```python
from build123d import *

# Parameters (mm, degrees)
F0_W     = 101.6
F0_H     = 50.8
F0_H_2   = 12.7
F0_H_3   = 76.2
F1_DEPTH = 12.7
F2_W     = 50.8
F2_H     = 203.2
F3_DEPTH = 25.4
F4_W     = 12.7
F4_H     = 50.8
F4_H_2   = 76.2
F5_DEPTH = 25.4
F6_W     = 139.7
F6_H     = 44.45
F7_DEPTH = 25.4


with BuildPart() as f1:
    # F0 (on Front) → F1 (new body)
    with BuildSketch(Plane.XZ):
        with Locations((-41.9671071525, -12.46464407)):
            Rectangle(F0_W, F0_H)
        with Locations((59.6328928475, -12.46464407)):
            Rectangle(F0_W, F0_H)
        with Locations((-41.9671071525, 139.93535593)):
            Rectangle(F0_W, F0_H)
        with Locations((59.6328928475, 139.93535593)):
            Rectangle(F0_W, F0_H)
        with Locations((-41.9671071525, 19.28535593)):
            Rectangle(F0_W, F0_H_2)
        with Locations((-41.9671071525, 63.73535593)):
            Rectangle(F0_W, F0_H_3)
        with Locations((-41.9671071525, 108.18535593)):
            Rectangle(F0_W, F0_H_2)
        with Locations((59.6328928475, 63.73535593)):
            Rectangle(F0_W, F0_H_3)
    extrude(amount=-F1_DEPTH)

    # F2 (on face) → F3 (cut)
    with BuildSketch(Plane.XZ):
        with Locations((85.0328928475, 63.73535593)):
            Rectangle(F2_W, F2_H)
    extrude(amount=-F3_DEPTH, mode=Mode.SUBTRACT)

    # F4 (on face) → F5 (cut)
    with BuildSketch(Plane.XZ):
        with Locations((53.2828928475, 139.93535593)):
            Rectangle(F4_W, F4_H)
        with Locations((53.2828928475, -12.46464407)):
            Rectangle(F4_W, F4_H)
        with Locations((53.2828928475, 63.73535593)):
            Rectangle(F4_W, F4_H_2)
    extrude(amount=-F5_DEPTH, mode=Mode.SUBTRACT)

    # F6 (on face) → F7 (cut)
    with BuildSketch(Plane.XZ):
        with Locations((-22.9171071525, 143.11035593)):
            Rectangle(F6_W, F6_H)
        with Locations((-22.9171071525, -15.63964407)):
            Rectangle(F6_W, F6_H)
    extrude(amount=-F7_DEPTH, mode=Mode.SUBTRACT)


solid = f1.part
```
Geometry: final body of the model. Coordinates: model frame, mm. A direction names the side the tool comes from. Coordinates: 2 decimals unless noted, no trailing zeros. Order: outer loops, then holes, each group sorted by start corner. A loop starts at its lowest first (then second) coordinate and runs counter-clockwise, first axis right, second up. Notation, with made-up numbers: M 22,-7 L 32,-7 A30 cw 32,27 Z; hole C -20,84.5 d11. An arc over 180 degrees is marked long. Answer in a Markdown table with one row per item. Add a question column.
Q1. Contact query for a flat-ended pin moving along its axis: P1, Ø4, axis at y = 9, z = 17.5, coming from the +X side. Output: stop coordinate, or through.
Q2. Line query: L1, parallel to Z at x = 11, y = 2; L2, parallel to X at y = 5, z = 19. Output: solid intervals per line, ascending.
Q3. Section query A-A on x = 27. Return the cut outline in (y, z), and give its area (3 significant figures).
Q4. Reachability of faces 4 (the flat face through (28, 6, 12.935)), 5 (the flat face through (46.933, 6, 118)) from +Z, -Z, +X, -X, +Y, -Y: full face, straight path, thin tool, end or side. Return the list, or none.
Q5. Mould query, pull axis Z, two halves, no side actions, for faces 1 (the flat face through (-24, 6, 120.885)), 2 (the flat face through (-24, 12.7, 65)), 3 (the flat face through (28, 6, 101.835)). Classes: released by +Z, released by -Z, zero draft, split by the parting line, or undercut.
Q6. Section query C-C on z = 105. Return the cut outline in (x, y), and give its area (3 significant figures).
Q7. Section query B-B on y = 2.25. Return the cut outline in (x, z).
Completed:
| question | item | result |
|---|---|---|
| 1 | P1 | stops at x = 8.83 |
| 2 | L1 | z = 6.59 to 12.94, 25.64 to 101.84, 114.54 to 120.89 |
| 2 | L2 | x = -92.77 to 8.83 |
| 3 | outline | M 0,6.59 L 12.7,6.59 L 12.7,12.94 L 0,12.94 Z; M 0,25.64 L 12.7,25.64 L 12.7,101.84 L 0,101.84 Z; M 0,114.54 L 12.7,114.54 L 12.7,120.89 L 0,120.89 Z |
| 3 | area | 1,130 mm2 |
| 4 | face 4 | +X, +Y, -Y |
| 4 | face 5 | +Z, -Z, +X, +Y, -Y |
| 5 | face 1 | released by +Z |
| 5 | face 2 | zero draft |
| 5 | face 3 | undercut |
| 6 | outline | M -92.77,0 L 8.83,0 L 8.83,12.7 L -92.77,12.7 Z |
| 6 | area | 1,290 mm2 |
| 7 | outline | M -92.77,6.59 L 46.93,6.59 L 46.93,12.94 L 8.83,12.94 L 8.83,25.64 L 46.93,25.64 L 46.93,101.84 L 8.83,101.84 L 8.83,114.54 L 46.93,114.54 L 46.93,120.89 L -92.77,120.89 Z |
